Could you check a few things on this model? Use its own coordinates, in mm. A direction names the side the tool comes from. Give positions to 0.01 mm unless a question says otherwise; leave off trailing zeros. Order: outer loops, then holes, each group sorted by start corner. A loop starts at its lowest first (then second) coordinate and runs counter-clockwise, first axis right, second up. Notation, with made-up numbers: (1, 20) -> (9, 20) arc R28 cw to (9, 54) -> close; hole circle Ø6 at (-4.75, 63). An arc over 180 degrees is marked (long way). Write each question's results on one line, items separated by ' | '.
```python
from build123d import *

# Parameters (mm, degrees)
SKETCH1_W               = 90
SKETCH1_H               = 64
BOSS_EXTRUDE1_DEPTH     = 23
SKETCH3_W               = 26
SKETCH3_H               = 9.317565448
CUT_EXTRUDE1_DEPTH      = 99.249681933
SKETCH4_W               = 28
SKETCH4_H               = 7.570604484
CUT_EXTRUDE2_DEPTH      = 82.547532152
BOSS_EXTRUDE2_DEPTH     = 64
CUT_EXTRUDE3_DEPTH      = 113.800709218
CUT_EXTRUDE3_DEPTH_BACK = 113.800709218
SKETCH7_W               = 8
SKETCH7_H               = 37
CUT_EXTRUDE4_DEPTH      = 113.800709218
CUT_EXTRUDE4_DEPTH_BACK = 113.800709218
SKETCH8_W               = 16
SKETCH8_H               = 25
CUT_EXTRUDE5_DEPTH      = 94.600213675
CUT_EXTRUDE5_DEPTH_BACK = 94.600213675
SKETCH9_R               = 20
SKETCH11_W              = 28
SKETCH11_H              = 15.933340455
CUT_EXTRUDE6_DEPTH      = 69.647220475


with BuildPart() as part:
    # Sketch1 → Boss-Extrude1 (new body)
    with BuildSketch(Plane(origin=(0, 0, 0), x_dir=(1, 0, 0), z_dir=(0, 1, 0))):
        Rectangle(SKETCH1_W, SKETCH1_H)
    extrude(amount=BOSS_EXTRUDE1_DEPTH)

    # Sketch3 → Cut-Extrude1 (cut, through all)
    with BuildSketch(Plane.ZY.offset(45)):
        Rectangle(SKETCH3_W, SKETCH3_H)
    extrude(amount=-CUT_EXTRUDE1_DEPTH, mode=Mode.SUBTRACT)

    # Sketch4 → Cut-Extrude2 (cut, through all)
    with BuildSketch(Plane.XY.offset(32)):
        with Locations((0, 23)):
            Rectangle(SKETCH4_W, SKETCH4_H)
    cut_extrude2 = extrude(amount=-CUT_EXTRUDE2_DEPTH, mode=Mode.SUBTRACT)

    # Sketch5 → Boss-Extrude2 (add, through all)
    with BuildSketch(Plane.XY.offset(32)):
        Polygon((-30, 60), (30, 60), (45, 23), (-45, 23), align=None)
    extrude(amount=-BOSS_EXTRUDE2_DEPTH)

    # Sketch7 → Cut-Extrude3 (cut, two sides: drawn at the far end of the back side and taken through both)
    with BuildSketch(Plane.ZY.offset(45).offset(-CUT_EXTRUDE3_DEPTH_BACK)):
        with Locations((-28, 41.5)):
            Rectangle(SKETCH7_W, SKETCH7_H)
        with Locations((28, 41.5)):
            Rectangle(SKETCH7_W, SKETCH7_H)
    extrude(amount=CUT_EXTRUDE3_DEPTH + CUT_EXTRUDE3_DEPTH_BACK, mode=Mode.SUBTRACT)

    # Sketch8 → Cut-Extrude4 (cut, two sides: drawn at the far end of the back side and taken through both)
    with BuildSketch(Plane.ZY.offset(45).offset(-CUT_EXTRUDE4_DEPTH_BACK)):
        with Locations((0, 47.5)):
            Rectangle(SKETCH8_W, SKETCH8_H)
    extrude(amount=CUT_EXTRUDE4_DEPTH + CUT_EXTRUDE4_DEPTH_BACK, mode=Mode.SUBTRACT)

    # Sketch9 → Cut-Extrude5 (cut, two sides: drawn at the far end of the back side and taken through both)
    with BuildSketch(Plane.XY.offset(24).offset(-CUT_EXTRUDE5_DEPTH_BACK)):
        with Locations((0, 60)):
            Circle(SKETCH9_R)
    extrude(amount=CUT_EXTRUDE5_DEPTH + CUT_EXTRUDE5_DEPTH_BACK, mode=Mode.SUBTRACT)

    # Sketch11 → Cut-Extrude6 (cut, through all)
    with BuildSketch(Plane(origin=(0, 19.214697758, 0), x_dir=(1, 0, 0), z_dir=(0, 1, 0))):
        with Locations((0, -24.033329773)):
            Rectangle(SKETCH11_W, SKETCH11_H)
    cut_extrude6 = extrude(amount=CUT_EXTRUDE6_DEPTH, mode=Mode.SUBTRACT)

    # Mirror1: Cut-Extrude2, Cut-Extrude6 across plane
    add(cut_extrude2.mirror(Plane.XY), mode=Mode.SUBTRACT)
    add(cut_extrude6.mirror(Plane.XY), mode=Mode.SUBTRACT)


solid = part.part
```
Q1. I'm going to push flat-ended pins straight in: pin 1 Ø12.5 at (x, y) = (3, 53) entering from +Z; pin 2 Ø4 at (x, z) = (-22.5, -27.5) entering from +Y; pin 3 Ø1 at (x, z) = (13, 25) entering from +Y; pin 4 Ø21 at (x, y) = (4.5, 40) entering from +Z. Where does each tip first touch, or does it pass through?
Here are the results:
pin 1: passes through | pin 2: stops at y = 23 | pin 3: stops at y = 19.21 | pin 4: stops at z = 24
Q2. Suppose I cut it at D-D on x = 27. Please give me the cut outline in (y, z), and give its area (3 significant figures).
Here are the results:
outline: (0, -32) -> (23, -32) -> (23, -24) -> (60, -24) -> (60, -8) -> (35, -8) -> (35, 8) -> (60, 8) -> (60, 24) -> (23, 24) -> (23, 32) -> (0, 32) -> (0, 13) -> (4.66, 13) -> (4.66, -13) -> (0, -13) -> close | area: 2,730 mm²
Q3. I need wall thicknesses on line 1 along Z through (x, y) = (21, 42.5); line 2 along Y through (x, z) = (-2, 0.5); line 3 along X through (y, z) = (21, -21.5). Which ranges of each line are inside material? Lowest first, please.
Here are the results:
line 1: z = -24 to -8, 8 to 24 | line 2: y = 4.66 to 19.21, 26.79 to 35 | line 3: x = -45 to -14, 14 to 45
Q4. Suppose I cut it at B-B on x = 0. Please give me the cut outline in (y, z), and give its area (3 significant figures).
Here are the results:
outline: (0, -32) -> (19.21, -32) -> (19.21, 32) -> (0, 32) -> (0, 13) -> (4.66, 13) -> (4.66, -13) -> (0, -13) -> close; (26.79, -16.07) -> (40, -16.07) -> (40, -8) -> (35, -8) -> (35, 8) -> (40, 8) -> (40, 16.07) -> (26.79, 16.07) -> close | area: 1,450 mm²
Q5. Suppose I cut it at C-C on z = 20. Please give me the cut outline in (x, y), and give its area (3 significant figures).
Here are the results:
outline: (-45, 0) -> (45, 0) -> (45, 23) -> (30, 60) -> (20, 60) arc R20 cw to (14, 45.72) -> (14, 19.21) -> (-14, 19.21) -> (-14, 45.72) arc R20 cw to (-20, 60) -> (-30, 60) -> (-45, 23) -> close | area: 3,580 mm²
Q6. Suppose I cut it at A-A on z = -14.5. Please give me the cut outline in (x, y).
Here are the results:
outline: (-45, 0) -> (45, 0) -> (45, 23) -> (30, 60) -> (20, 60) arc R20 cw to (-20, 60) -> (-30, 60) -> (-45, 23) -> close; hole (-14, 19.21) -> (14, 19.21) -> (14, 26.79) -> (-14, 26.79) -> close
Q7. For faces 1 (the cylindrical face through (0, 40, -14)), 2 (the flat face through (-29, 23, -28)), 3 (the flat face through (-14, 26, 0)), 4 (the flat face through (26, 37, 24)), 5 (the flat face through (0, 26.785, 0)), which set-ups out of +Z, -Z, +X, -X, +Y, -Y let a thin tool reach every point of the face, with its end or its side?
Here are the results:
face 1: +Z, -Z, +Y | face 2: -Z, +X, -X, +Y | face 3: none | face 4: +Z, +X, -X, +Y | face 5: +Z, -Z
Q8. Thinking about a two-plate mould opening in X: for faces 6 (the flat face through (14, 26, 0)), 7 (the flat face through (25, 60, -16)), 8 (the flat face through (40.728, 33.537, 0.336)), which applies, +X half, -X half, draft (parallel to the pull), parting line (faces both ways), or undercut?
Here are the results:
face 6: undercut | face 7: draft | face 8: +X half
